Autodesk Inventor part; units mm, degrees
ref_plane "YZ Plane" through (0, 0, 0) normal (1, 0, 0) x (0, 1, 0)
ref_plane "XZ Plane" through (0, 0, 0) normal (0, 1, 0) x (-1, 0, 0)
ref_plane "XY Plane" through (0, 0, 0) normal (0, 0, 1) x (1, 0, 0)
sketch "Boceto39" plane through (0, 0, 0) normal (0, 0, 1) x (1, 0, 0)
  line L0 (-24, 6.25) -> (24, 6.25)
  line L1 (24, 6.25) -> (24, -6.25)
  line L2 (24, -6.25) -> (-24, -6.25)
  line L3 (-24, -6.25) -> (-24, 6.25)
  point P0 (0, 0)
  point P1 (0, 6.25)
  point P2 (-24, 0)
  dimension "d373" = 48
  dimension "d374" = 12.5
extrude "Extrusión13" add sketch "Boceto39" along normal blind 12.5
sketch "Boceto40" plane through (0, 0, 0) normal (0, 1, 0) x (-1, 0, 0)
  line L0 (24, 0) -> (-24, 0)
  line L1 (24, 0) -> (24, 12.5)
  line L2 (-24, 12.5) -> (24, 12.5)
  line L3 (-24, 0) -> (-24, 12.5)
  line L4 (-27, -4.2347) -> (-27, 4.25)
  line L5 (-25, 6.25) -> (25, 6.25)
  line L6 (27, 4.25) -> (27, -6)
  arc A0 (27, 4.25) -> (25, 6.25) centre (25, 4.25) ccw
  arc A1 (-25, 6.25) -> (-27, 4.25) centre (-25, 4.25) ccw
  point P0 (0, 0)
  point P1 (0, 6.25)
  point P2 (24, 6.25)
  point P3 (0, 0)
  dimension "d377" = 27
  dimension "d378" = 2
  dimension "d379" = 6
sketch "Boceto41" plane through (0, 0, 0) normal (1, 0, 0) x (0, 1, 0)
  circle A0 centre (0, 6.25) radius 0.4
  point P0 (0, 0)
  dimension "d380" = 0.8
sweep "Barrido1" add profiles "Boceto41" path "Boceto40" path curves L6 A0 L5 A1 L4
properties part number "AXIAL-POWER-5W"
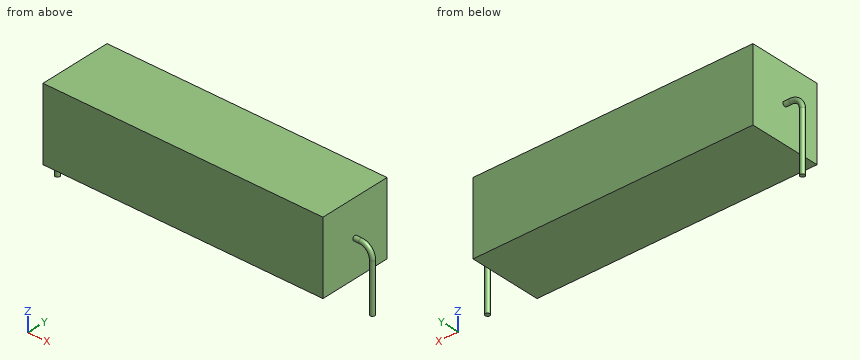
Design review of the part built by this model. Coordinates are the model's own, in mm. Give positions to 0.01 mm unless a question says otherwise; leave off trailing zeros. Loops run counter-clockwise (first coordinate to the right, second up) from the corner with the lowest first, then second, coordinate; pieces in that order, holes last. Notation, with made-up numbers: (60.25, -26.75) -> (113.25, -26.75) arc R15 ccw to (113.25, -15.75) -> close; hole circle Ø3 at (-22.75, -29). An arc over 180 degrees is marked (long way). One line per item, written item: value.
Q1. For pin 1 Ø4 at (y, z) = (-3, 8.5) entering from +X; pin 2 Ø4 at (y, z) = (-1, 6.5) entering from -X; pin 3 Ø1.5 at (x, y) = (4, 1) entering from -Z; pin 4 Ø6 at (y, z) = (0.5, 4) entering from +X, all flat-tipped, find the tip position at first contact; note any pin that passes through.
Numbers:
pin 1: stops at x = 24
pin 2: stops at x = -27.35
pin 3: stops at z = 0
pin 4: stops at x = 27.4
Q2. We need section B-B on y = 1.75. Give the boundary of the cut face in (x, z).
Numbers:
outline: (-24, 0) -> (24, 0) -> (24, 12.5) -> (-24, 12.5) -> close
Q3. We need section A-A on z = -2. Give the boundary of the cut face in (x, y).
Numbers:
outline: circle Ø0.8 at (-27, 0); circle Ø0.8 at (27, 0)
Q4. We need section C-C on z = 9.5. Give the boundary of the cut face in (x, y), and give its area (3 significant figures).
Numbers:
outline: (-24, -6.25) -> (24, -6.25) -> (24, 6.25) -> (-24, 6.25) -> close
area: 600 mm^2
Q5. For L1, parallel to Z at x = 5.5, y = -1.5; L2, parallel to X at y = 1.75, z = 3.75; L3, parallel to X at y = 0, z = -2, list the stretches that pass through material, from the lowest coordinate up.
Numbers:
L1: z = 0 to 12.5
L2: x = -24 to 24
L3: x = -27.4 to -26.6, 26.6 to 27.4
